Model file for the job. Use its own axes, mm. Face numbers are marked on the shaded views. A direction names the side the tool comes from. Round coordinates to 2 decimals unless told otherwise and drop trailing zeros. Order: outer loops, then holes, each group sorted by start corner. A loop starts at its lowest first (then second) coordinate and runs counter-clockwise, first axis right, second up. Notation, with made-up numbers: (34.5, -37.75) - (66.5, -37.75) arc R27 ccw to (66.5, -14.75) - close; hole circle Ø8 at (-15.5, 32.5). An arc over 180 degrees is marked (long way). Answer as CSV lines item,"result". Start each with the question number.
1. Band-saw the part on C-C on y = -8.5. List the corners of the cut face in (x, z), then the cut area to 3 significant figures.
2. Band-saw the part on B-B on x = 0. List the corners of the cut face in (y, z).
3. Pin check, flat tips, straight feed: pin 1 Ø7 at (x, y) = (13.98, -16.66) entering from -Z; pin 2 Ø1.5 at (y, z) = (-20.5, 2.5) entering from -X; pin 3 Ø1.5 at (x, z) = (-1.5, 6) entering from -Y. Stop position of each tip, or through.
4. Wall check: line 1 along Y through (x, z) = (-13, 4.5); line 2 along X through (y, z) = (1.5, 4.6); line 3 along X through (y, z) = (16, 2.1). Give the ranges that are in metal, low to high. Write a range as [from, to].
5. Pull direction X, two halves, no side cores. Call the marked faces 1, 2 and 3: released by +X, released by -X, zero draft, split by the parting line, or undercut.
6. 3-axis set-ups, long thin cutter, end or side, ignore diameter. For the marked faces 4 and 5: which of +Z, -Z, +X, -X, +Y, -Y reach the whole face in a straight line?
7. Band-saw the part on A-A on y = 0. List the corners of the cut face in (x, z).
8. Band-saw the part on D-D on z = 2.2. List the corners of the cut face in (x, y), then the cut area to 3 significant figures.
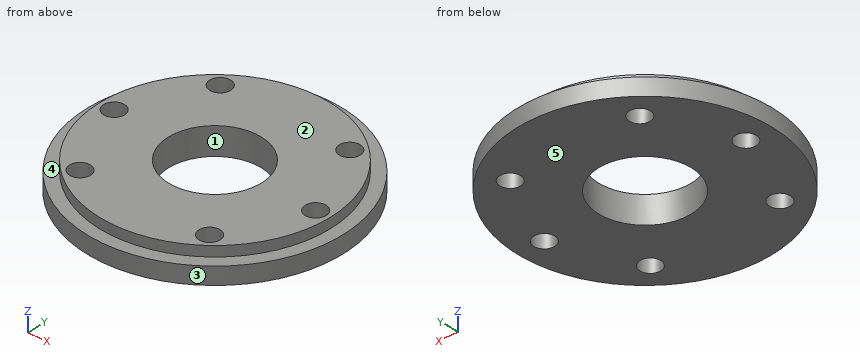
```python
from build123d import *

# Parameters (mm, degrees)
SKETCH_1_R          = 24.85
SKETCH_1_R_2        = 2.25
EXTRUDE_1_DEPTH     = 6.5
SKETCH_3_R          = 27.5
SKETCH_3_R_2        = 24.85
EXTRUDE_2_DEPTH     = 4.3
SKETCH_4_R          = 27.5
CUT_EXTRUDE_1_DEPTH = 0.6
SKETCH_5_R          = 10
CUT_EXTRUDE_2_DEPTH = 40.335861501


with BuildPart() as part:
    # 草图1 → 凸台-拉伸1 (new body)
    with BuildSketch(Plane.XY):
        with Locations(Location((0, 0, 0), (0, 0, 180))):
            Circle(SKETCH_1_R)
        with Locations(Location((-21.75, 0, 0), (0, 0, 180))):
            Circle(SKETCH_1_R_2, mode=Mode.SUBTRACT)
        with Locations(Location((-13.980630511, 16.661466638, 0), (0, 0, 180))):
            Circle(SKETCH_1_R_2, mode=Mode.SUBTRACT)
        with Locations(Location((-13.980630511, -16.661466638, 0), (0, 0, 180))):
            Circle(SKETCH_1_R_2, mode=Mode.SUBTRACT)
        with Locations(Location((13.980630511, -16.661466638, 0), (0, 0, 180))):
            Circle(SKETCH_1_R_2, mode=Mode.SUBTRACT)
        with Locations(Location((21.75, 0, 0), (0, 0, 180))):
            Circle(SKETCH_1_R_2, mode=Mode.SUBTRACT)
        with Locations(Location((13.980630511, 16.661466638, 0), (0, 0, 180))):
            Circle(SKETCH_1_R_2, mode=Mode.SUBTRACT)
    extrude(amount=EXTRUDE_1_DEPTH)

    # 草图3 → 凸台-拉伸2 (add)
    with BuildSketch(Plane.XY):
        with Locations(Location((0, 0, 0), (0, 0, 180))):
            Circle(SKETCH_3_R)
        with Locations(Location((0, 0, 0), (0, 0, 180))):
            Circle(SKETCH_3_R_2, mode=Mode.SUBTRACT)
    extrude(amount=EXTRUDE_2_DEPTH)

    # 草图4 → 切除-拉伸1 (cut)
    with BuildSketch(Plane(origin=(0, 0, 0), x_dir=(-1, 0, 0), z_dir=(0, 0, -1))):
        Circle(SKETCH_4_R)
    extrude(amount=-CUT_EXTRUDE_1_DEPTH, mode=Mode.SUBTRACT)

    # 草图5 → 切除-拉伸2 (cut, through all)
    with BuildSketch(Plane(origin=(0, 0, 0.6), x_dir=(-1, 0, 0), z_dir=(0, 0, -1))):
        Circle(SKETCH_5_R)
    extrude(amount=-CUT_EXTRUDE_2_DEPTH, mode=Mode.SUBTRACT)


solid = part.part
```
Reply:
1,outline,"(-26.15, 0.6) - (-5.27, 0.6) - (-5.27, 6.5) - (-23.35, 6.5) - (-23.35, 4.3) - (-26.15, 4.3) - close; (5.27, 0.6) - (26.15, 0.6) - (26.15, 4.3) - (23.35, 4.3) - (23.35, 6.5) - (5.27, 6.5) - close"
1,area,"234 mm2"
2,outline,"(-27.5, 0.6) - (-10, 0.6) - (-10, 6.5) - (-24.85, 6.5) - (-24.85, 4.3) - (-27.5, 4.3) - close; (10, 0.6) - (27.5, 0.6) - (27.5, 4.3) - (24.85, 4.3) - (24.85, 6.5) - (10, 6.5) - close"
3,pin 1,"stops at z = 0.6"
3,pin 2,"stops at x = -19.14"
3,pin 3,"stops at y = -24.84"
4,line 1,"y = [-21.18, -18.69], [-14.64, 14.64], [18.69, 21.18]"
4,line 2,"x = [-24.8, -23.43], [-20.07, -9.89], [9.89, 20.07], [23.43, 24.8]"
4,line 3,"x = [-22.37, -16.13], [-11.83, 11.83], [16.13, 22.37]"
5,face 1,"undercut"
5,face 2,"zero draft"
5,face 3,"split by the parting line"
6,face 4,"+Z"
6,face 5,"-Z, +X, -X, +Y, -Y"
7,outline,"(-27.5, 0.6) - (-24, 0.6) - (-24, 6.5) - (-24.85, 6.5) - (-24.85, 4.3) - (-27.5, 4.3) - close; (-19.5, 0.6) - (-10, 0.6) - (-10, 6.5) - (-19.5, 6.5) - close; (10, 0.6) - (19.5, 0.6) - (19.5, 6.5) - (10, 6.5) - close; (24, 0.6) - (27.5, 0.6) - (27.5, 4.3) - (24.85, 4.3) - (24.85, 6.5) - (24, 6.5) - close"
8,outline,"circle Ø55 at (0, 0); hole circle Ø4.5 at (-21.75, 0); hole circle Ø4.5 at (-13.98, -16.66); hole circle Ø4.5 at (-13.98, 16.66); hole circle Ø20 at (0, 0); hole circle Ø4.5 at (13.98, -16.66); hole circle Ø4.5 at (13.98, 16.66); hole circle Ø4.5 at (21.75, 0)"
8,area,"1,970 mm2"
